```python
from build123d import *

# Parameters (mm, degrees)
BOSS_EXTRUDE1_DEPTH  = 12.7
SKETCH2_R            = 4.7625
CUT_EXTRUDE1_DEPTH   = 3.175
SHELL2_START         = 6.35
SHELL2_DEPTH         = 6.35
FILLET3_R            = 6.35
BOSS_EXTRUDE2_DEPTH  = 6.35
CUT_EXTRUDE2_START   = 6.35
SKETCH4_W            = 25.908
SKETCH4_H            = 10.922
CUT_EXTRUDE2_DEPTH   = 2.032
CUT_EXTRUDE3_DEPTH   = 6.35
SKETCH6_R            = 31.75
SKETCH6_R_2          = 25.4
BOSS_EXTRUDE3_DEPTH  = 2.54
SKETCH7_R            = 19.05
SKETCH7_R_2          = 12.7
BOSS_EXTRUDE4_DEPTH  = 2.54
SKETCH8_R            = 6.35
SKETCH8_R_2          = 3.175
BOSS_EXTRUDE5_DEPTH  = 2.54
BOSS_EXTRUDE6_DEPTH  = 2.54
LPATTERN1_COUNT      = 2
LPATTERN1_PITCH      = 15.24
MIRROR3_COPY_1_DEPTH = 2.54


# Read off the part's stored shape, not the designer's step: Shell2
with BuildPart() as part:
    # Sketch1 → Boss-Extrude1 (new body)
    with BuildSketch(Plane(origin=(0, 0, 0), x_dir=(1, 0, 0), z_dir=(0, 1, 0))):
        Polygon((-76.2, 44.45), (-101.6, 19.05), (-101.6, -19.05), (-76.2, -44.45), (76.2, -44.45), (101.6, -19.05), (101.6, 19.05), (76.2, 44.45), align=None)
    extrude(amount=BOSS_EXTRUDE1_DEPTH)

    # Sketch2 → Cut-Extrude1 (cut)
    with BuildSketch(Plane(origin=(0, 12.7, 0), x_dir=(1, 0, 0), z_dir=(0, 1, 0))):
        with Locations(Location((-63.5, -38.608, 0), (0, 0, 270))):
            Circle(SKETCH2_R)
    cut_extrude1 = extrude(amount=-CUT_EXTRUDE1_DEPTH, mode=Mode.SUBTRACT)

    # Mirror1: Cut-Extrude1 across plane
    add(cut_extrude1.mirror(Plane(origin=(0, 0, 0), x_dir=(0, 0, 1), z_dir=(1, 0, 0))), mode=Mode.SUBTRACT)

    # Shell2 outline → Shell2 (cut)
    with BuildSketch(Plane(origin=(0, 0, 0), x_dir=(1, 0, 0), z_dir=(0, 1, 0)).offset(SHELL2_START)):
        with BuildLine():
            Line((74.516823481, -37.152920398), (95.25, -16.419743879))
            Line((95.25, -16.419743879), (95.25, 16.419743879))
            Line((95.25, 16.419743879), (73.569743879, 38.1))
            Line((73.569743879, 38.1), (-73.569743879, 38.1))
            Line((-73.569743879, 38.1), (-95.25, 16.419743879))
            Line((-95.25, 16.419743879), (-95.25, -16.419743879))
            Line((-95.25, -16.419743879), (-74.516823481, -37.152920398))
            ThreePointArc((-74.516823481, -37.152920398), (-63.024598672, -27.505673675), (-52.399117501, -38.1))
            Line((-52.399117501, -38.1), (52.399117501, -38.1))
            ThreePointArc((52.399117501, -38.1), (63.024598672, -27.505673675), (74.516823481, -37.152920398))
        make_face()
    extrude(amount=SHELL2_DEPTH, mode=Mode.SUBTRACT)

    # Fillet3
    fillet3_edges = [part.edges().sort_by_distance(p)[0] for p in [
        (95.25, 9.525, 16.419743879),
        (95.25, 9.525, -16.419743879),
        (73.569743879, 9.525, -38.1),
        (-73.569743879, 9.525, -38.1),
        (-95.25, 9.525, -16.419743879),
        (-95.25, 9.525, 16.419743879),
        (52.399117501, 9.525, 38.1),
        (-52.399117501, 9.525, 38.1),
        (-74.516823481, 9.525, 37.152920398),
        (74.516823481, 9.525, 37.152920398),
    ]]
    fillet(fillet3_edges, radius=FILLET3_R)

    # Sketch3 → Boss-Extrude2 (add)
    with BuildSketch(Plane(origin=(0, 6.35, 0), x_dir=(1, 0, 0), z_dir=(0, 1, 0))):
        Polygon((-76.2, 44.45), (-63.5, 31.75), (63.5, 31.75), (76.2, 44.45), align=None)
    extrude(amount=BOSS_EXTRUDE2_DEPTH)

    # Sketch4 → Cut-Extrude2 (cut)
    with BuildSketch(Plane(origin=(0, 6.35, 0), x_dir=(1, 0, 0), z_dir=(0, 1, 0)).offset(CUT_EXTRUDE2_START)):
        with Locations((-50.8, 38.989)):
            Rectangle(SKETCH4_W, SKETCH4_H)
    cut_extrude2 = extrude(amount=-CUT_EXTRUDE2_DEPTH, mode=Mode.SUBTRACT)

    # Mirror2: Cut-Extrude2 across plane
    add(cut_extrude2.mirror(Plane(origin=(0, 0, 0), x_dir=(0, 0, 1), z_dir=(1, 0, 0))), mode=Mode.SUBTRACT)

    # Sketch5 → Cut-Extrude3 (cut)
    with BuildSketch(Plane(origin=(0, 12.7, 0), x_dir=(1, 0, 0), z_dir=(0, 1, 0))):
        Polygon((-37.846, 31.75), (-31.496, 38.1), (31.496, 38.1), (37.846, 31.75), align=None)
    extrude(amount=-CUT_EXTRUDE3_DEPTH, mode=Mode.SUBTRACT)

    # Sketch6 → Boss-Extrude3 (add)
    with BuildSketch(Plane(origin=(0, 6.35, 0), x_dir=(1, 0, 0), z_dir=(0, 1, 0))):
        with Locations(Location((0, 0, 0), (0, 0, 270))):
            Circle(SKETCH6_R)
        with Locations(Location((0, 0, 0), (0, 0, 270))):
            Circle(SKETCH6_R_2, mode=Mode.SUBTRACT)
    extrude(amount=BOSS_EXTRUDE3_DEPTH)

    # Sketch7 → Boss-Extrude4 (add)
    with BuildSketch(Plane(origin=(0, 6.35, 0), x_dir=(1, 0, 0), z_dir=(0, 1, 0))):
        with Locations(Location((0, 0, 0), (0, 0, 270))):
            Circle(SKETCH7_R)
        with Locations(Location((0, 0, 0), (0, 0, 270))):
            Circle(SKETCH7_R_2, mode=Mode.SUBTRACT)
    extrude(amount=BOSS_EXTRUDE4_DEPTH)

    # Sketch8 → Boss-Extrude5 (add)
    with BuildSketch(Plane(origin=(0, 6.35, 0), x_dir=(1, 0, 0), z_dir=(0, 1, 0))):
        with Locations(Location((0, 0, 0), (0, 0, 270))):
            Circle(SKETCH8_R)
        with Locations(Location((0, 0, 0), (0, 0, 270))):
            Circle(SKETCH8_R_2, mode=Mode.SUBTRACT)
    extrude(amount=BOSS_EXTRUDE5_DEPTH)

    # Sketch9 → Boss-Extrude6 (add)
    with BuildSketch(Plane(origin=(0, 6.35, 0), x_dir=(1, 0, 0), z_dir=(0, 1, 0))):
        with BuildLine():
            ThreePointArc((-38.494829198, 22.225), (-44.45, 0), (-38.494829198, -22.225))
            ThreePointArc((-38.494829198, -22.225), (-34.157698541, -23.387130657), (-32.995567884, -19.05))
            ThreePointArc((-32.995567884, -19.05), (-38.1, 0), (-32.995567884, 19.05))
            ThreePointArc((-32.995567884, 19.05), (-34.157698541, 23.387130657), (-38.494829198, 22.225))
        make_face()
    boss_extrude6 = extrude(amount=BOSS_EXTRUDE6_DEPTH)

    # LPattern1: Boss-Extrude6 ×2
    with Locations(*[(-i * LPATTERN1_PITCH, 0, 0) for i in range(1, LPATTERN1_COUNT)]):
        add(boss_extrude6)

    # Mirror3: Boss-Extrude6 across plane
    add(boss_extrude6.mirror(Plane(origin=(0, 0, 0), x_dir=(0, 0, 1), z_dir=(1, 0, 0))))

    # Mirror3 copy 1 sketch → Mirror3 copy 1 (add)
    with BuildSketch(Plane(origin=(15.24, 6.35, 0), x_dir=(-1, 0, 0), z_dir=(0, 1, 0))):
        with BuildLine():
            ThreePointArc((-38.494829198, -22.225), (-44.45, 0), (-38.494829198, 22.225))
            ThreePointArc((-38.494829198, 22.225), (-34.157698541, 23.387130657), (-32.995567884, 19.05))
            ThreePointArc((-32.995567884, 19.05), (-38.1, 0), (-32.995567884, -19.05))
            ThreePointArc((-32.995567884, -19.05), (-34.157698541, -23.387130657), (-38.494829198, -22.225))
        make_face()
    extrude(amount=MIRROR3_COPY_1_DEPTH)


solid = part.part
```
Design review of the part built by this model. Coordinates are the model's own, in mm. A direction names the side the tool comes from. Coordinates: 2 decimals unless noted, no trailing zeros. Loops run counter-clockwise (first coordinate to the right, second up) from the corner with the lowest first, then second, coordinate; pieces in that order, holes last. Notation, with made-up numbers: M 7,77 L 63,77 A30 ccw 63,102 Z; hole C 6.5,-24.5 d10. An arc over 180 degrees is marked long. One line per question, with ' | ' between items.
(1) Wall thickness on probe 1 along Z at (x, y) = (-40, 9.5); probe 2 along X at (y, z) = (9.25, -35.5); probe 3 along Y at (x, z) = (-76, -24.5): over which ranges is each line inside the solid? List them lowest first.
Filled in:
probe 1: z = -44.45 to -31.75, 38.1 to 44.45 | probe 2: x = -85.15 to -76.17, -67.25 to -34.1, 34.1 to 67.25, 76.17 to 85.15 | probe 3: y = 0 to 6.35
(2) We need section C-C (x = -87.5). Give the boundary of the cut face in (y, z).
Filled in:
outline: M 0,-33.15 L 12.7,-33.15 L 12.7,-24.17 L 6.35,-24.17 L 6.35,24.17 L 12.7,24.17 L 12.7,33.15 L 0,33.15 Z
(3) We need section B-B (x = 27.5). Give the boundary of the cut face in (y, z).
Filled in:
outline: M 0,-44.45 L 12.7,-44.45 L 12.7,-38.1 L 6.35,-38.1 L 6.35,-15.87 L 8.89,-15.87 L 8.89,15.87 L 6.35,15.87 L 6.35,38.1 L 12.7,38.1 L 12.7,44.45 L 0,44.45 Z
(4) Draft analysis for pull direction Z (two halves, no side actions). For faces 1 (the face through (53.34, 7.6, 0.28)), 2 (the face through (-51, 10.668, -39)), state which applies: released by +Z, released by -Z, zero draft, split by the parting line, or undercut.
Filled in:
face 1: undercut | face 2: zero draft
(5) For pin 1 Ø3.5 at (x, z) = (39, -8.5) entering from +Y; pin 2 Ø1 at (x, y) = (53.5, 12) entering from -Z; pin 3 Ø5 at (x, z) = (65, 38.5) entering from +Y (3 decimals), all flat-tipped, find the tip position at first contact; note any pin that passes through.
Filled in:
pin 1: stops at y = 8.89 | pin 2: stops at z = -33.53 | pin 3: stops at y = 9.525
(6) Machinability: for faces 3 (the face through (-101.6, 6, 0)), 4 (the face through (-54, 8.89, 0)), which of the approach directions +Z, -Z, +X, -X, +Y, -Y give a long, thin tool a straight path to every point of the face, cutting with its end or side? Answer none if there is none.
Filled in:
face 3: +Z, -Z, -X, +Y, -Y | face 4: +Y
